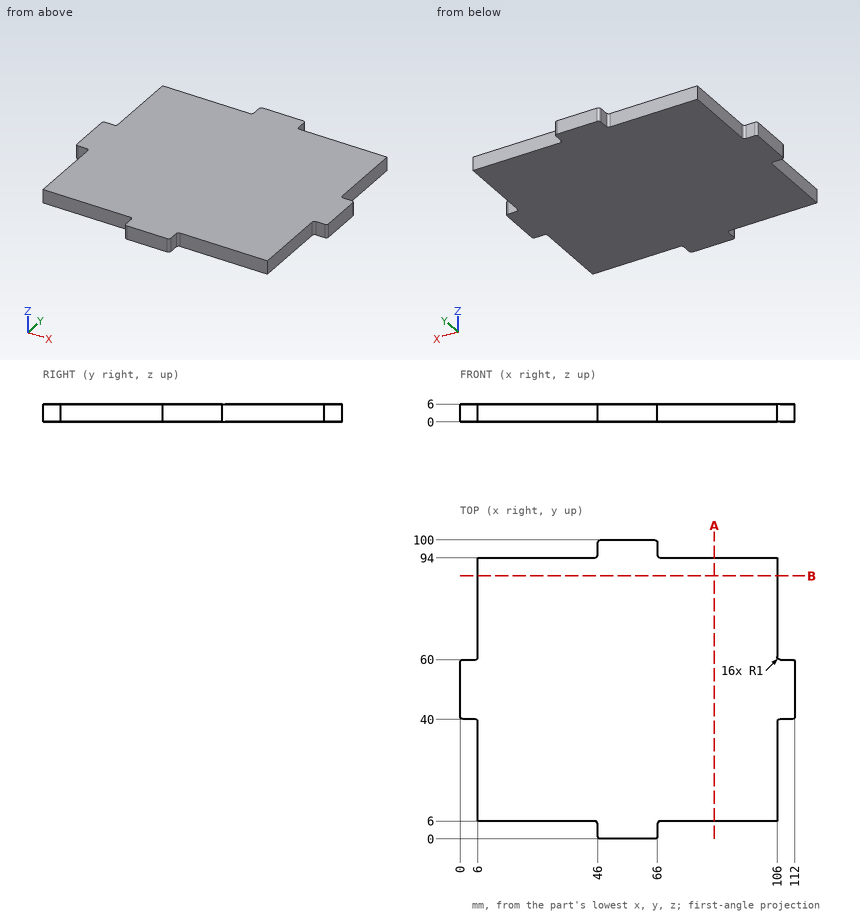
Source: three-view drawing plus pictorial views. Frame: mm from the lowest corner of the part. Round coordinates to 2 decimals unless told otherwise and drop trailing zeros. Loops run counter-clockwise (first coordinate to the right, second up) from the corner with the lowest first, then second, coordinate; pieces in that order, holes last.
Q1. Ray query, line 1 (Y direction, x = 101, z = 2.7); line 2 (X direction, y = 93, z = 5.7); line 3 (X direction, y = 39.5, z = 2). Return the intervals inside material, ascending.
Q2. Section B-B, the plane y = 88. Return loops of the section in (x, z).
Q3. Section A-A, the plane x = 85. Return loops of the section in (y, z).
Q4. First-contact query: P1, Ø1.5, axis at x = 34, z = 2, coming from the +Y side; P2, Ø8, axis at x = 50.5, y = 38, coming from the -Z side; P3, Ø1.2, axis at x = 109, z = 2, coming from the -Y side; P4, Ø1.8, axis at y = 70.5, z = 3, coming from the +X side. Flat tips, straight axial feed; report the tip coordinate or a pass-through.
Solutions:
1. line 1: y = 6 to 94
1. line 2: x = 6 to 106
1. line 3: x = 5.87 to 106.13
2. outline: (6, 0) - (106, 0) - (106, 6) - (6, 6) - close
3. outline: (6, 0) - (94, 0) - (94, 6) - (6, 6) - close
4. P1: stops at y = 94
4. P2: stops at z = 0
4. P3: stops at y = 40
4. P4: stops at x = 106
